Part print with two shaded views. Sizes in mm from the minimum x, y, z corner. A direction names the side the tool comes from. Coordinates: 2 decimals unless noted, no trailing zeros. Order: outer loops, then holes, each group sorted by start corner. A loop starts at its lowest first (then second) coordinate and runs counter-clockwise, first axis right, second up. Notation, with made-up numbers: (62, 35.25) - (73, 35.25) arc R32 cw to (73, 61.25) - close; hole circle Ø5 at (63, 70.25). An arc over 180 degrees is marked (long way). Return JSON: item names as keys, results as strings.
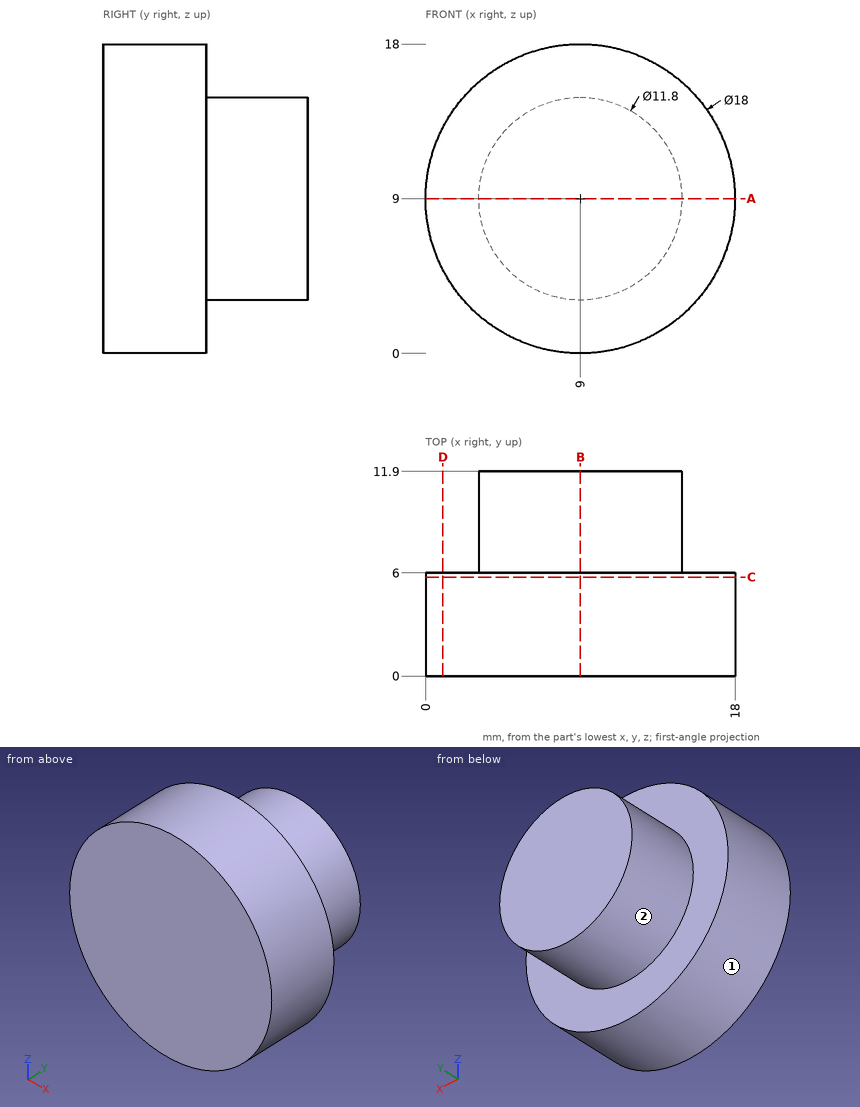
Item 1: Band-saw the part on A-A, the plane z = 9. List the corners of the cut face in (x, y).
Findings below:
{"outline": "(0, 0) - (18, 0) - (18, 6) - (14.9, 6) - (14.9, 11.9) - (3.1, 11.9) - (3.1, 6) - (0, 6) - close"}
Item 2: Wall check: L1, parallel to Y at x = 1.5, z = 9.5; L2, parallel to Z at x = 8, y = 3.25; L3, parallel to Z at x = 5, y = 8. Give the ranges that are in metal, low to high. Write a range as [from, to].
Findings below:
{"L1": "y = [0, 6]", "L2": "z = [0.06, 17.94]", "L3": "z = [4.66, 13.34]"}
Item 3: Band-saw the part on D-D, the plane x = 1. List the corners of the cut face in (y, z).
Findings below:
{"outline": "(0, 4.88) - (6, 4.88) - (6, 13.12) - (0, 13.12) - close"}
Item 4: Band-saw the part on C-C, the plane y = 5.75. List the corners of the cut face in (x, z), then the cut area to 3 significant figures.
Findings below:
{"outline": "circle Ø18 at (9, 9)", "area": "254 mm²"}
Item 5: Which spindle directions (+Z, -Z, +X, -X, +Y, -Y) get a long thin tool onto all of the face, cutting with end or side? Do the marked faces 1 and 2. Say none if no direction does.
Findings below:
{"face 1": "+Y, -Y", "face 2": "+Y"}
Item 6: Drop flat-ended pins along their axis: P1, Ø1.5, axis at x = 13.5, y = 3, coming from the +Z side; P2, Ø1, axis at x = 7.5, z = 16, coming from the +Y side; P3, Ø4, axis at x = 10, y = 9, coming from the +Z side. Give the stop position or say it passes through.
Findings below:
{"P1": "stops at z = 17.18", "P2": "stops at y = 6", "P3": "stops at z = 14.9"}
Item 7: Band-saw the part on B-B, the plane x = 9. List the corners of the cut face in (y, z).
Findings below:
{"outline": "(0, 0) - (6, 0) - (6, 3.1) - (11.9, 3.1) - (11.9, 14.9) - (6, 14.9) - (6, 18) - (0, 18) - close"}
